Could you check a few things on this model? Use its own coordinates, in mm. Round coordinates to 2 decimals unless told otherwise and drop trailing zeros. Write each loop counter-clockwise with the first axis right and the second up, starting at its lowest first coordinate (ties: lowest second). Pieces come first, ordered by that corner, then holes. Notation, with made-up numbers: (70, 35.5) -> (77, 35.5) arc R37 ccw to (77, 72.5) -> close; hole circle Ø7 at (88, 34.25). An arc over 180 degrees is marked (long way). Answer in a Markdown table with one row per item. Add a question column.
```python
from build123d import *

# Parameters (mm, degrees)
F1_DEPTH = 6.35
F3_DEPTH = 12.7
F5_DEPTH = 25.4


with BuildPart() as f1:
    # F0 (on Top) → F1 (new body)
    with BuildSketch(Plane.XY):
        with BuildLine():
            ThreePointArc((0, 19.05), (5.579616, 5.579616), (19.05, 0))
            Line((19.05, 0), (209.55, 0))
            ThreePointArc((209.55, 0), (223.020384, 5.579616), (228.6, 19.05))
            Line((228.6, 19.05), (228.6, 50.8))
            Line((228.6, 50.8), (0, 50.8))
            Line((0, 50.8), (0, 19.05))
        make_face()
    extrude(amount=F1_DEPTH)

    # F2 (on face) → F3 (join)
    with BuildSketch(Plane.XY.offset(6.35)):
        with BuildLine():
            Line((12.7, 50.8), (12.7, 19.05))
            ThreePointArc((12.7, 19.05), (14.559872, 14.559872), (19.05, 12.7))
            Line((19.05, 12.7), (209.55, 12.7))
            ThreePointArc((209.55, 12.7), (214.040128, 14.559872), (215.9, 19.05))
            Line((215.9, 19.05), (215.9, 50.8))
            Line((215.9, 50.8), (12.7, 50.8))
        make_face()
    extrude(amount=F3_DEPTH)

    # F4 (on face) → F5 (cut)
    with BuildSketch(Plane.XY.offset(19.05)):
        with BuildLine():
            ThreePointArc((29.36875, 50.8), (25.4, 54.76875), (21.43125, 50.8))
            Line((21.43125, 50.8), (29.36875, 50.8))
        make_face()
        with BuildLine():
            Line((29.36875, 50.8), (21.43125, 50.8))
            ThreePointArc((21.43125, 50.8), (25.4, 46.83125), (29.36875, 50.8))
        make_face()
        with BuildLine():
            ThreePointArc((54.76875, 50.8), (50.8, 54.76875), (46.83125, 50.8))
            Line((46.83125, 50.8), (54.76875, 50.8))
        make_face()
        with BuildLine():
            Line((54.76875, 50.8), (46.83125, 50.8))
            ThreePointArc((46.83125, 50.8), (50.8, 46.83125), (54.76875, 50.8))
        make_face()
        with BuildLine():
            ThreePointArc((72.23125, 50.8), (76.2, 46.83125), (80.16875, 50.8))
            Line((80.16875, 50.8), (72.23125, 50.8))
        make_face()
        with BuildLine():
            ThreePointArc((199.23125, 50.8), (203.2, 46.83125), (207.16875, 50.8))
            Line((207.16875, 50.8), (199.23125, 50.8))
        make_face()
        with BuildLine():
            ThreePointArc((173.83125, 50.8), (177.8, 46.83125), (181.76875, 50.8))
            Line((181.76875, 50.8), (173.83125, 50.8))
        make_face()
        with BuildLine():
            ThreePointArc((148.43125, 50.8), (152.4, 46.83125), (156.36875, 50.8))
            Line((156.36875, 50.8), (148.43125, 50.8))
        make_face()
        with BuildLine():
            ThreePointArc((123.03125, 50.8), (127, 46.83125), (130.96875, 50.8))
            Line((130.96875, 50.8), (123.03125, 50.8))
        make_face()
        with BuildLine():
            Line((97.63125, 50.8), (105.56875, 50.8))
            ThreePointArc((105.56875, 50.8), (101.6, 54.76875), (97.63125, 50.8))
        make_face()
        with BuildLine():
            Line((72.23125, 50.8), (80.16875, 50.8))
            ThreePointArc((80.16875, 50.8), (76.2, 54.76875), (72.23125, 50.8))
        make_face()
        with BuildLine():
            Line((199.23125, 50.8), (207.16875, 50.8))
            ThreePointArc((207.16875, 50.8), (203.2, 54.76875), (199.23125, 50.8))
        make_face()
        with BuildLine():
            Line((173.83125, 50.8), (181.76875, 50.8))
            ThreePointArc((181.76875, 50.8), (177.8, 54.76875), (173.83125, 50.8))
        make_face()
        with BuildLine():
            Line((148.43125, 50.8), (156.36875, 50.8))
            ThreePointArc((156.36875, 50.8), (152.4, 54.76875), (148.43125, 50.8))
        make_face()
        with BuildLine():
            Line((123.03125, 50.8), (130.96875, 50.8))
            ThreePointArc((130.96875, 50.8), (127, 54.76875), (123.03125, 50.8))
        make_face()
        with BuildLine():
            ThreePointArc((97.63125, 50.8), (101.6, 46.83125), (105.56875, 50.8))
            Line((105.56875, 50.8), (97.63125, 50.8))
        make_face()
    extrude(amount=-F5_DEPTH, mode=Mode.SUBTRACT)


solid = f1.part
```
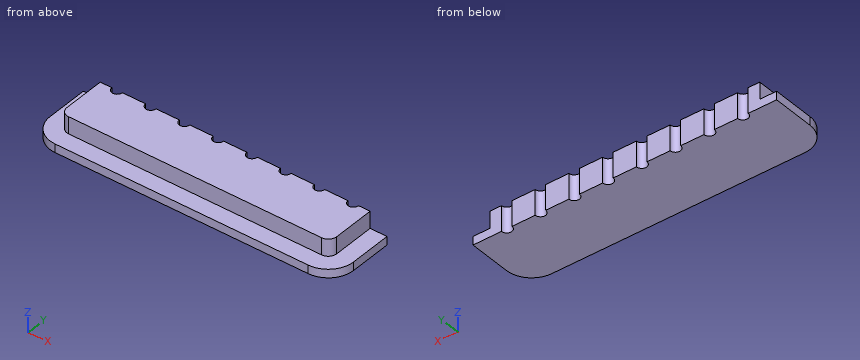
(1) Suppose I cut it at A-A, the plane y = 39. Please give me the cut outline in (x, z), then the cut area to 3 significant figures.
(2) I need wall thicknesses on L1, parallel to X at y = 46.5, z = 10.75; L2, parallel to Z at x = 61.5, y = 9; L3, parallel to Y at x = 45, z = 16.75. Which ranges of each line are inside material? Lowest first, please.
(3) Suppose I cut it at B-B, the plane z = 12. Please give me the cut outline in (x, y).
(4) Suppose I cut it at D-D, the plane y = 17. Please give me the cut outline in (x, z).
(5) Suppose I cut it at C-C, the plane x = 25.4. Please give me the cut outline in (y, z), then the cut area to 3 significant figures.
(6) For P1, Ø6.5, axis at y = 31.5, z = 14.5, coming from the +X side; P2, Ø6.5, axis at x = 86.5, z = 15, coming from the -Y side; P3, Ø1.5, axis at y = 42, z = 16, coming from the -X side, each with a flat end and sliding along its axis, tell me the tip position at first contact or that it passes through.
Response:
| question | item | result |
|---|---|---|
| 1 | outline | (0, 0) -> (228.6, 0) -> (228.6, 6.35) -> (215.9, 6.35) -> (215.9, 19.05) -> (12.7, 19.05) -> (12.7, 6.35) -> (0, 6.35) -> close |
| 1 | area | 4,030 mm² |
| 2 | L1 | 12.7 to 215.9 |
| 2 | L2 | 0 to 6.35 |
| 2 | L3 | 12.7 to 50.8 |
| 3 | outline | (12.7, 19.05) arc R6.35 ccw to (19.05, 12.7) -> (209.55, 12.7) arc R6.35 ccw to (215.9, 19.05) -> (215.9, 50.8) -> (207.17, 50.8) arc R3.97 cw to (199.23, 50.8) -> (181.77, 50.8) arc R3.97 cw to (173.83, 50.8) -> (156.37, 50.8) arc R3.97 cw to (148.43, 50.8) -> (130.97, 50.8) arc R3.97 cw to (123.03, 50.8) -> (105.57, 50.8) arc R3.97 cw to (97.63, 50.8) -> (80.17, 50.8) arc R3.97 cw to (72.23, 50.8) -> (54.77, 50.8) arc R3.97 cw to (46.83, 50.8) -> (29.37, 50.8) arc R3.97 cw to (21.43, 50.8) -> (12.7, 50.8) -> close |
| 4 | outline | (0.11, 0) -> (228.49, 0) -> (228.49, 6.35) -> (215.56, 6.35) -> (215.56, 19.05) -> (13.04, 19.05) -> (13.04, 6.35) -> (0.11, 6.35) -> close |
| 5 | outline | (0, 0) -> (46.83, 0) -> (46.83, 19.05) -> (12.7, 19.05) -> (12.7, 6.35) -> (0, 6.35) -> close |
| 5 | area | 731 mm² |
| 6 | P1 | x = 215.9 |
| 6 | P2 | y = 12.7 |
| 6 | P3 | x = 12.7 |
